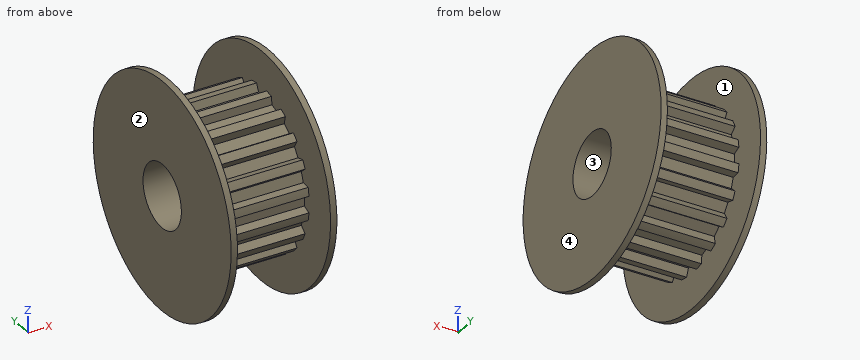
from build123d import *

# Parameters (mm, degrees)
SKETCH1_W                    = 0.5
SKETCH1_H                    = 9
BOSS_EXTRUDE1_DEPTH          = 7.4
SKETCH3_R                    = 9
BOSS_EXTRUDE2_DEPTH          = 0.5
F_5_0_5_DIAMETER_HOLE1_D     = 5
F_5_0_5_DIAMETER_HOLE1_DEPTH = 8.4


with BuildPart() as part:
    # Sketch1 → Revolve1 (revolve)
    with BuildSketch(Plane(origin=(0, 0, 0), x_dir=(-1, 0, 0), z_dir=(0, 0, -1))):
        with Locations((-7.65, 4.5)):
            Rectangle(SKETCH1_W, SKETCH1_H)
    revolve(axis=Axis((7.9, 0, 0), (-1, 0, 0)))

    # Sketch2 → Boss-Extrude1 (add)
    with BuildSketch(Plane.ZY.offset(-7.4)):
        with BuildLine():
            Line((6.078441347, -1.295675803), (5.437383609, -1.346128141))
            Line((5.437383609, -1.346128141), (5.190170014, -2.106973354))
            Line((5.190170014, -2.106973354), (5.679141478, -2.524594437))
            ThreePointArc((5.679141478, -2.524594437), (5.537605548, -2.821550956), (5.38055541, -3.110602591))
            Line((5.38055541, -3.110602591), (4.755282641, -2.96048788))
            Line((4.755282641, -2.96048788), (4.285054439, -3.607701476))
            Line((4.285054439, -3.607701476), (4.621041925, -4.155983221))
            ThreePointArc((4.621041925, -4.155983221), (4.394668645, -4.394668645), (4.155983221, -4.621041925))
            Line((4.155983221, -4.621041925), (3.607701476, -4.285054439))
            Line((3.607701476, -4.285054439), (2.96048788, -4.755282641))
            Line((2.96048788, -4.755282641), (3.110602591, -5.38055541))
            ThreePointArc((3.110602591, -5.38055541), (2.821550956, -5.537605548), (2.524594437, -5.679141478))
            Line((2.524594437, -5.679141478), (2.106973354, -5.190170014))
            Line((2.106973354, -5.190170014), (1.346128141, -5.437383609))
            Line((1.346128141, -5.437383609), (1.295675803, -6.078441347))
            ThreePointArc((1.295675803, -6.078441347), (0.9722402, -6.138483037), (0.64608076, -6.181327095))
            Line((0.64608076, -6.181327095), (0.4, -5.587235585))
            Line((0.4, -5.587235585), (-0.4, -5.587235585))
            Line((-0.4, -5.587235585), (-0.64608076, -6.181327095))
            ThreePointArc((-0.64608076, -6.181327095), (-0.9722402, -6.138483037), (-1.295675803, -6.078441347))
            Line((-1.295675803, -6.078441347), (-1.346128141, -5.437383609))
            Line((-1.346128141, -5.437383609), (-2.106973354, -5.190170014))
            Line((-2.106973354, -5.190170014), (-2.524594437, -5.679141478))
            ThreePointArc((-2.524594437, -5.679141478), (-2.821550956, -5.537605548), (-3.110602591, -5.38055541))
            Line((-3.110602591, -5.38055541), (-2.96048788, -4.755282641))
            Line((-2.96048788, -4.755282641), (-3.607701476, -4.285054439))
            Line((-3.607701476, -4.285054439), (-4.155983221, -4.621041925))
            ThreePointArc((-4.155983221, -4.621041925), (-4.394668645, -4.394668645), (-4.621041925, -4.155983221))
            Line((-4.621041925, -4.155983221), (-4.285054439, -3.607701476))
            Line((-4.285054439, -3.607701476), (-4.755282641, -2.96048788))
            Line((-4.755282641, -2.96048788), (-5.38055541, -3.110602591))
            ThreePointArc((-5.38055541, -3.110602591), (-5.537605548, -2.821550956), (-5.679141478, -2.524594437))
            Line((-5.679141478, -2.524594437), (-5.190170014, -2.106973354))
            Line((-5.190170014, -2.106973354), (-5.437383609, -1.346128141))
            Line((-5.437383609, -1.346128141), (-6.078441347, -1.295675803))
            ThreePointArc((-6.078441347, -1.295675803), (-6.138483037, -0.9722402), (-6.181327095, -0.64608076))
            Line((-6.181327095, -0.64608076), (-5.587235585, -0.4))
            Line((-5.587235585, -0.4), (-5.587235585, 0.4))
            Line((-5.587235585, 0.4), (-6.181327095, 0.64608076))
            ThreePointArc((-6.181327095, 0.64608076), (-6.138483037, 0.9722402), (-6.078441347, 1.295675803))
            Line((-6.078441347, 1.295675803), (-5.437383609, 1.346128141))
            Line((-5.437383609, 1.346128141), (-5.190170014, 2.106973354))
            Line((-5.190170014, 2.106973354), (-5.679141478, 2.524594437))
            ThreePointArc((-5.679141478, 2.524594437), (-5.537605548, 2.821550956), (-5.38055541, 3.110602591))
            Line((-5.38055541, 3.110602591), (-4.755282641, 2.96048788))
            Line((-4.755282641, 2.96048788), (-4.285054439, 3.607701476))
            Line((-4.285054439, 3.607701476), (-4.621041925, 4.155983221))
            ThreePointArc((-4.621041925, 4.155983221), (-4.394668645, 4.394668645), (-4.155983221, 4.621041925))
            Line((-4.155983221, 4.621041925), (-3.607701476, 4.285054439))
            Line((-3.607701476, 4.285054439), (-2.96048788, 4.755282641))
            Line((-2.96048788, 4.755282641), (-3.110602591, 5.38055541))
            ThreePointArc((-3.110602591, 5.38055541), (-2.821550956, 5.537605548), (-2.524594437, 5.679141478))
            Line((-2.524594437, 5.679141478), (-2.106973354, 5.190170014))
            Line((-2.106973354, 5.190170014), (-1.346128141, 5.437383609))
            Line((-1.346128141, 5.437383609), (-1.295675803, 6.078441347))
            ThreePointArc((-1.295675803, 6.078441347), (-0.9722402, 6.138483037), (-0.64608076, 6.181327095))
            Line((-0.64608076, 6.181327095), (-0.4, 5.587235585))
            Line((-0.4, 5.587235585), (0.4, 5.587235585))
            Line((0.4, 5.587235585), (0.64608076, 6.181327095))
            ThreePointArc((0.64608076, 6.181327095), (0.9722402, 6.138483037), (1.295675803, 6.078441347))
            Line((1.295675803, 6.078441347), (1.346128141, 5.437383609))
            Line((1.346128141, 5.437383609), (2.106973354, 5.190170014))
            Line((2.106973354, 5.190170014), (2.524594437, 5.679141478))
            ThreePointArc((2.524594437, 5.679141478), (2.821550956, 5.537605548), (3.110602591, 5.38055541))
            Line((3.110602591, 5.38055541), (2.96048788, 4.755282641))
            Line((2.96048788, 4.755282641), (3.607701476, 4.285054439))
            Line((3.607701476, 4.285054439), (4.155983221, 4.621041925))
            ThreePointArc((4.155983221, 4.621041925), (4.394668645, 4.394668645), (4.621041925, 4.155983221))
            Line((4.621041925, 4.155983221), (4.285054439, 3.607701476))
            Line((4.285054439, 3.607701476), (4.755282641, 2.96048788))
            Line((4.755282641, 2.96048788), (5.38055541, 3.110602591))
            ThreePointArc((5.38055541, 3.110602591), (5.537605548, 2.821550956), (5.679141478, 2.524594437))
            Line((5.679141478, 2.524594437), (5.190170014, 2.106973354))
            Line((5.190170014, 2.106973354), (5.437383609, 1.346128141))
            Line((5.437383609, 1.346128141), (6.078441347, 1.295675803))
            ThreePointArc((6.078441347, 1.295675803), (6.138483037, 0.9722402), (6.181327095, 0.64608076))
            Line((6.181327095, 0.64608076), (5.587235585, 0.4))
            Line((5.587235585, 0.4), (5.587235585, -0.4))
            Line((5.587235585, -0.4), (6.181327095, -0.64608076))
            ThreePointArc((6.181327095, -0.64608076), (6.138483037, -0.9722402), (6.078441347, -1.295675803))
        make_face()
    extrude(amount=BOSS_EXTRUDE1_DEPTH)

    # Sketch3 → Boss-Extrude2 (add)
    with BuildSketch(Plane(origin=(0, 0, 0), x_dir=(0, 0, -1), z_dir=(1, 0, 0))):
        Circle(SKETCH3_R)
    extrude(amount=-BOSS_EXTRUDE2_DEPTH)

    # Ø5.0 (5) Diameter Hole1
    with Locations(Plane(origin=(7.9, 0, 0), x_dir=(0, 0, -1), z_dir=(1, 0, 0))):
        with Locations((0, 0)):
            Hole(F_5_0_5_DIAMETER_HOLE1_D / 2, depth=F_5_0_5_DIAMETER_HOLE1_DEPTH)


solid = part.part
Read the model definition and answer for the solid it produces. Units are mm, in the model's axes. Face numbers are marked on the shaded views. A direction names the side the tool comes from. Give positions to 0.01 mm unless a question says otherwise; leave off trailing zeros. Write each loop counter-clockwise with the first axis right and the second up, starting at its lowest first coordinate (ties: lowest second). Pieces come first, ordered by that corner, then holes. Notation, with made-up numbers: (-15, 0) - (36, 0) arc R24 cw to (36, 23) - close; hole circle Ø2 at (-7.5, -11.75). An arc over 180 degrees is marked (long way). Return JSON: item names as keys, results as strings.
Q1. Given P1, Ø0.9, axis at x = 2.5, y = 0, coming from the +Z side; P2, Ø0.9, axis at x = 4, z = 0, coming from the -Y side; P3, Ø3, axis at y = 0, z = 0, coming from the +X side; P4, Ø1, axis at x = 7, z = -1, coming from the +Y side, each flat-ended and moving along its own axis, determine where each tip first touches the part or whether it passes through.
Reply:
{"P1": "z = 5.71", "P2": "y = -5.71", "P3": "through", "P4": "y = 8.97"}
Q2. For a pull along Z with two mould halves and no side action, classify the marked faces 3 and 4 as released by +Z, released by -Z, zero draft, split by the parting line, or undercut.
Reply:
{"face 3": "undercut", "face 4": "zero draft"}
Q3. For the marked faces 1 and 2, determine the directions among +Z, -Z, +X, -X, +Y, -Y from which every point of the face is accessible in a straight line to the end or side of a thin tool.
Reply:
{"face 1": "none", "face 2": "+Z, -Z, -X, +Y, -Y"}
Q4. A cutting plane is placed at C-C, the plane y = 6.5. Determine the outline of the cut face in (x, z), and give its area (3 significant figures).
Reply:
{"outline": "(-0.5, -6.22) - (0, -6.22) - (0, 6.22) - (-0.5, 6.22) - close; (7.4, -6.22) - (7.9, -6.22) - (7.9, 6.22) - (7.4, 6.22) - close", "area": "12.4 mm²"}
Q5. A cutting plane is placed at A-A, the plane y = 0. Determine the outline of the cut face in (x, z).
Reply:
{"outline": "(-0.5, -9) - (0, -9) - (0, -5.59) - (7.4, -5.59) - (7.4, -9) - (7.9, -9) - (7.9, -2.5) - (-0.5, -2.5) - close; (-0.5, 2.5) - (7.9, 2.5) - (7.9, 9) - (7.4, 9) - (7.4, 5.59) - (0, 5.59) - (0, 9) - (-0.5, 9) - close"}
Q6. Consider line 1 along Y through (x, z) = (2.75, 0); line 2 along X through (y, z) = (-1, 6.75); line 3 along Z through (x, y) = (6.25, -0.25). Determine where each line is inside the solid, lowest interval first. Write a range as [from, to].
Reply:
{"line 1": "[-5.59, -2.5], [2.5, 5.59]", "line 2": "[-0.5, 0], [7.4, 7.9]", "line 3": "[-5.59, -2.49], [2.49, 5.59]"}
